Here's the drawing with two shaded views (mm, measured from the low corner). I have some questions. A direction names the side the tool comes from. Give positions to 0.01 mm unless a question says otherwise; leave off trailing zeros. Loops run counter-clockwise (first coordinate to the right, second up) from the corner with the lowest first, then second, coordinate; pieces in that order, holes last. Notation, with made-up numbers: M -4,-4 L 43,-4 A24 cw 43,20 Z; hole C -33.5,82 d8. An arc over 180 degrees is marked long. Put each result on its own line as item: value. Start each with the question number.
1) Imagine slicing it at C-C (z = 36). Write out the boundary of the cut face in (x, y).
2) Imagine slicing it at B-B (y = 15). Write out the boundary of the cut face in (x, z).
3) Imagine slicing it at A-A (x = 30). Write out the boundary of the cut face in (y, z).
4) If we mould it in two halves opening along X, with no side actions, what happens to the marked faces 3, 4, 5 and 6? For each: +X half, -X half, draft (parallel to the pull), parting line (faces both ways), or undercut.
5) Please list where these lines run through material, in increasing order: line 1 along X through (y, z) = (15.5, 58); line 2 along Z through (x, y) = (13, 17); line 3 along Y through (x, z) = (30, 39.5). Write a range as from..to.
6) Imagine slicing it at D-D (x = 36). Write out the boundary of the cut face in (y, z).
7) For the marked faces 1 and 2, which set-ups out of +Z, -Z, +X, -X, +Y, -Y let a thin tool reach every point of the face, with its end or its side?
8) For P1, Ø1, axis at x = 22, y = 3, coming from the -Z side; P2, Ø7, axis at y = 21.5, z = 86, coming from the +X side; P3, Ø12, axis at x = 23.5, y = 13, coming from the +Z side; P4, Ø12, axis at y = 25.5, z = 66.5, coming from the -X side, each with a flat end and sliding along its axis, tell me the tip position at first contact or that it passes through.
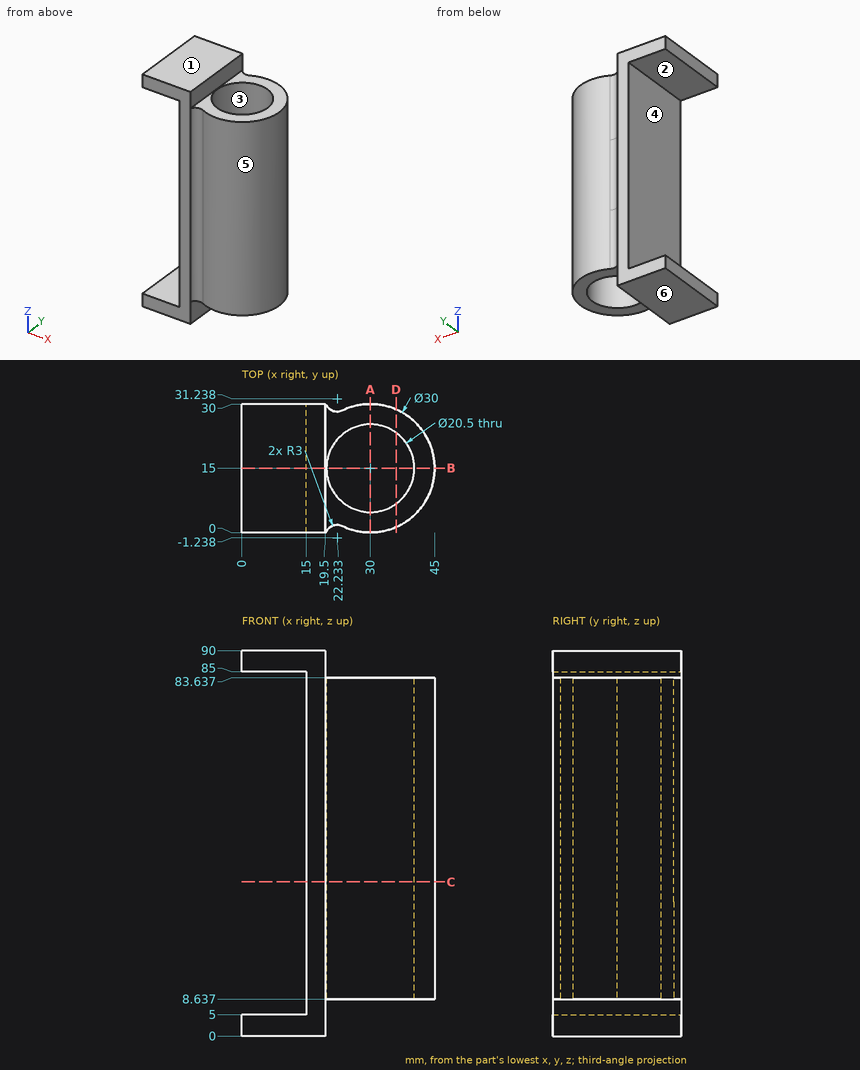
Recorded:
1. outline: M 15,0 L 19.5,0 A3 cw 23.53,1.47 A15 ccw long 23.53,28.53 A3 cw 19.5,30 L 15,30 Z; hole C 30,15 d20.5
2. outline: M 0,0 L 19.5,0 L 19.5,8.64 L 19.75,8.64 L 19.75,83.64 L 19.5,83.64 L 19.5,90 L 0,90 L 0,85 L 15,85 L 15,5 L 0,5 Z; M 40.25,8.64 L 45,8.64 L 45,83.64 L 40.25,83.64 Z
3. outline: M 0,8.64 L 4.75,8.64 L 4.75,83.64 L 0,83.64 Z; M 25.25,8.64 L 30,8.64 L 30,83.64 L 25.25,83.64 Z
4. face 3: undercut
4. face 4: -X half
4. face 5: undercut
4. face 6: draft
5. line 1: 15..19.76, 40.24..44.99
5. line 2: 0..5, 85..90
5. line 3: 0..4.75, 25.25..30
6. outline: M 1.25,8.64 L 6.69,8.64 L 6.69,83.64 L 1.25,83.64 Z; M 23.31,8.64 L 28.75,8.64 L 28.75,83.64 L 23.31,83.64 Z
7. face 1: +Z, +X, -X, +Y, -Y
7. face 2: -X, +Y, -Y
8. P1: z = 8.64
8. P2: x = 44.48
8. P3: z = 90
8. P4: x = 15
